Design review of the part built by this model. Coordinates are the model's own, in mm. Round coordinates to 2 decimals unless told otherwise and drop trailing zeros. Order: outer loops, then holes, each group sorted by start corner. A loop starts at its lowest first (then second) coordinate and runs counter-clockwise, first axis right, second up. Notation, with made-up numbers: (68.25, -30) - (88.25, -30) arc R27 ccw to (88.25, 5) - close; hole circle Ø5 at (78, 28.5). An arc over 180 degrees is marked (long way). Use CSV: the item, a comma, the result in double quotes.
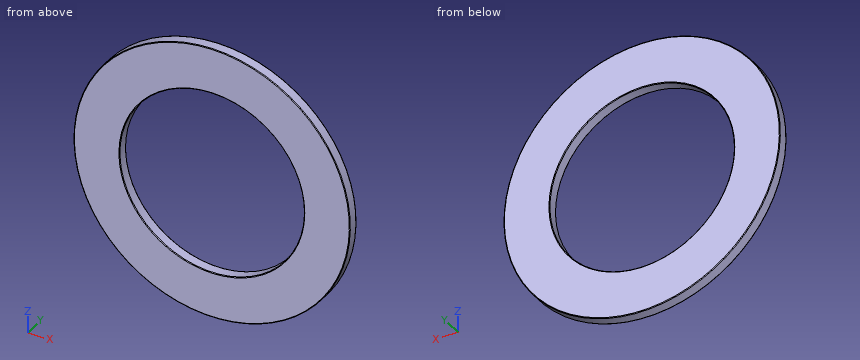
from build123d import *

# Parameters (mm, degrees)
SKETCH4_W = 7.8994
SKETCH4_H = 1.849966709
FILLET3_R = 0.110998


with BuildPart() as part:
    # Sketch4 → Revolve3 (revolve)
    with BuildSketch(Plane(origin=(0, 0, 0), x_dir=(0, 0, -1), z_dir=(1, 0, 0))):
        with Locations((-19.8628, -4.624916645)):
            Rectangle(SKETCH4_W, SKETCH4_H)
    revolve(axis=Axis((0, -5.5499, 0), (0, 1, 0)))

    # Fillet3
    fillet3_edges = [part.edges().sort_by_distance(p)[0] for p in [
        (0, -5.5499, -23.8125),
        (0, -5.5499, -15.9131),
        (0, -3.699933291, -15.9131),
        (0, -3.699933291, -23.8125),
    ]]
    fillet(fillet3_edges, radius=FILLET3_R)


solid = part.part
1) We need section B-B (y = -4.1). Give the boundary of the cut face in (x, z) (1 decimal), then the cut area to 3 significant figures.
Data:
outline,"circle Ø47.6 at (0, 0); hole circle Ø31.8 at (0, 0)"
area,"986 mm2"
2) To check wall thickness, follow L1, parallel to X at y = -4.6, z = 0; L2, parallel to Z at x = -7, y = -3.75; L3, parallel to Z at x = 10, y = -5.35. State the ranges of each line that lie inside material, in increasing order. Write a range as from..to.
Data:
L1,"x = -23.81..-15.91, 15.91..23.81"
L2,"z = -22.74..-14.31, 14.31..22.74"
L3,"z = -21.61..-12.38, 12.38..21.61"
3) We need section A-A (z = 0). Give the boundary of the cut face in (x, y).
Data:
outline,"(-23.81, -5.44) arc R0.11 ccw to (-23.7, -5.55) - (-16.02, -5.55) arc R0.11 ccw to (-15.91, -5.44) - (-15.91, -3.81) arc R0.11 ccw to (-16.02, -3.7) - (-23.7, -3.7) arc R0.11 ccw to (-23.81, -3.81) - close; (15.91, -5.44) arc R0.11 ccw to (16.02, -5.55) - (23.7, -5.55) arc R0.11 ccw to (23.81, -5.44) - (23.81, -3.81) arc R0.11 ccw to (23.7, -3.7) - (16.02, -3.7) arc R0.11 ccw to (15.91, -3.81) - close"
4) Insertion check: pin 1 Ø19 at (x, z) = (0, 0) entering from +Y. The pin has a flat end and moves straight along its axis. Give the tip position at first contact, or say it passes through.
Data:
pin 1,"passes through"
